Build history of the part. All positions in model axes, mm. Round coordinates to 2 decimals unless told otherwise and drop trailing zeros. Loops run counter-clockwise (first coordinate to the right, second up) from the corner with the lowest first, then second, coordinate; pieces in that order, holes last.
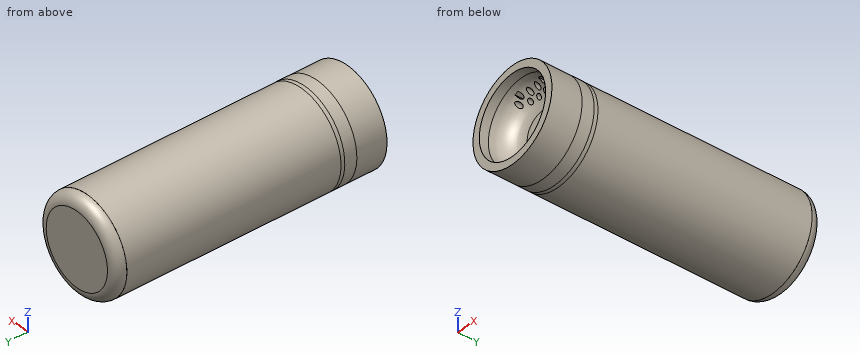
from build123d import *

# Parameters (mm, degrees)
SKETCH1_R           = 15.591175954
BOSS_EXTRUDE1_DEPTH = 71
BOSS_EXTRUDE2_START = 1.25
SKETCH2_R           = 15.591175954
SKETCH2_W           = 17.8
SKETCH2_H           = 1.65
BOSS_EXTRUDE2_DEPTH = 1.25
BOSS_EXTRUDE3_START = 4
SKETCH3_R           = 15.591175954
BOSS_EXTRUDE3_DEPTH = 4
CUT_EXTRUDE4_START  = -11.5
SKETCH16_R          = 0.75
CUT_EXTRUDE4_DEPTH  = 11.5
BOSS_EXTRUDE8_START = 10
SKETCH18_R          = 15.591175954
SKETCH18_R_2        = 13.095738675
BOSS_EXTRUDE8_DEPTH = 10
FILLET3_START       = -12.2500001
FILLET3_OUTLINE_R   = 13.095738675
FILLET3_OUTLINE_R_2 = 0.75
FILLET3_DEPTH       = 7.0000001
FILLET3_START_2     = -11
FILLET3_3_DEPTH     = 5.75
SKETCH26_R          = 15.591175954
BOSS_EXTRUDE9_DEPTH = 3.5
FILLET4_R           = 3.5


with BuildPart() as part:
    # Sketch1 → Boss-Extrude1 (new body)
    with BuildSketch(Plane(origin=(0, 0, 0), x_dir=(1, 0, 0), z_dir=(0, 1, 0))):
        with Locations(Location((0, 0, 0), (0, 0, 270))):
            Circle(SKETCH1_R)
        with BuildLine():
            Line((8.375, -6.964282891), (9.075, -6.964282891))
            Line((9.075, -6.964282891), (9.075, -8.614282891))
            Line((9.075, -8.614282891), (8.375, -8.614282891))
            Line((8.375, -8.614282891), (8.375, -9.610929808))
            ThreePointArc((8.375, -9.610929808), (0, -12.747964417), (-8.375, -9.610929808))
            Line((-8.375, -9.610929808), (-8.375, -8.614282891))
            Line((-8.375, -8.614282891), (-8.725, -8.614282891))
            Line((-8.725, -8.614282891), (-8.725, -6.964282891))
            Line((-8.725, -6.964282891), (-8.375, -6.964282891))
            Line((-8.375, -6.964282891), (-8.375, -6.204282891))
            Line((-8.375, -6.204282891), (-8.375, 9.645717109))
            ThreePointArc((-8.375, 9.645717109), (-7.386485387, 12.032202496), (-5, 13.020717109))
            Line((-5, 13.020717109), (5, 13.020717109))
            ThreePointArc((5, 13.020717109), (7.386485387, 12.032202496), (8.375, 9.645717109))
            Line((8.375, 9.645717109), (8.375, -6.204282891))
            Line((8.375, -6.204282891), (8.375, -6.964282891))
        make_face(mode=Mode.SUBTRACT)
    extrude(amount=BOSS_EXTRUDE1_DEPTH)

    # Sketch2 → Boss-Extrude2 (add)
    with BuildSketch(Plane.XZ.offset(BOSS_EXTRUDE2_START)):
        with Locations(Location((0, 0, 0), (0, 0, 270))):
            Circle(SKETCH2_R)
        with Locations((0.175, 7.789282891)):
            Rectangle(SKETCH2_W, SKETCH2_H, mode=Mode.SUBTRACT)
    extrude(amount=-BOSS_EXTRUDE2_DEPTH)

    # Sketch3 → Boss-Extrude3 (add)
    with BuildSketch(Plane.XZ.offset(1.25).offset(BOSS_EXTRUDE3_START)):
        with Locations(Location((0, 0, 0), (0, 0, 270))):
            Circle(SKETCH3_R)
    extrude(amount=-BOSS_EXTRUDE3_DEPTH)

    # Sketch16 → Cut-Extrude4 (cut)
    with BuildSketch(Plane(origin=(0, 0, 0), x_dir=(1, 0, 0), z_dir=(0, 1, 0)).offset(CUT_EXTRUDE4_START)):
        with BuildLine():
            Line((-3.75, -9.901070776), (-3, -9.901070776))
            Line((-3, -9.901070776), (-2.25, -9.901070776))
            ThreePointArc((-2.25, -9.901070776), (-3, -9.151070776), (-3.75, -9.901070776))
        make_face()
        with BuildLine():
            Line((-2.25, -9.901070776), (-3, -9.901070776))
            Line((-3, -9.901070776), (-3.75, -9.901070776))
            ThreePointArc((-3.75, -9.901070776), (-3, -10.651070776), (-2.25, -9.901070776))
        make_face()
        with BuildLine():
            ThreePointArc((6.75, -9.901070776), (6, -9.151070776), (5.25, -9.901070776))
            ThreePointArc((5.25, -9.901070776), (6, -10.651070776), (6.75, -9.901070776))
        make_face()
        with BuildLine():
            ThreePointArc((3.75, -9.901070776), (3, -9.151070776), (2.25, -9.901070776))
            Line((2.25, -9.901070776), (3, -9.901070776))
            Line((3, -9.901070776), (3.75, -9.901070776))
        make_face()
        with BuildLine():
            Line((3, -9.901070776), (2.25, -9.901070776))
            ThreePointArc((2.25, -9.901070776), (3, -10.651070776), (3.75, -9.901070776))
            Line((3.75, -9.901070776), (3, -9.901070776))
        make_face()
        with BuildLine():
            ThreePointArc((0.75, -9.901070776), (0, -9.151070776), (-0.75, -9.901070776))
            Line((-0.75, -9.901070776), (0, -9.901070776))
            Line((0, -9.901070776), (0.75, -9.901070776))
        make_face()
        with BuildLine():
            Line((0, -9.901070776), (-0.75, -9.901070776))
            ThreePointArc((-0.75, -9.901070776), (0, -10.651070776), (0.75, -9.901070776))
            Line((0.75, -9.901070776), (0, -9.901070776))
        make_face()
        with Locations(Location((-6, -9.901070776, 0), (0, 0, 270))):
            Circle(SKETCH16_R)
        with BuildLine():
            ThreePointArc((5.289192257, -11.598924176), (4.550417773, -10.824582592), (3.789595018, -11.577272013))
            ThreePointArc((3.789595018, -11.577272013), (3.846450326, -11.860961254), (4.006459728, -12.102019552))
            ThreePointArc((4.006459728, -12.102019552), (4.654628095, -11.867815051), (5.289192257, -11.598924176))
        make_face()
        with BuildLine():
            ThreePointArc((2.290136401, -11.577272013), (1.540136401, -10.827272013), (0.790136401, -11.577272013))
            Line((0.790136401, -11.577272013), (1.540136401, -11.577272013))
            Line((1.540136401, -11.577272013), (2.290136401, -11.577272013))
        make_face()
        with BuildLine():
            Line((1.540136401, -11.577272013), (0.790136401, -11.577272013))
            ThreePointArc((0.790136401, -11.577272013), (1.540136401, -12.327272013), (2.290136401, -11.577272013))
            Line((2.290136401, -11.577272013), (1.540136401, -11.577272013))
        make_face()
        with BuildLine():
            ThreePointArc((-0.707561207, -11.577133163), (-2.207561203, -11.577063737), (-0.707561219, -11.577272013))
            ThreePointArc((-0.707561219, -11.577272013), (-0.70756121, -11.577202588), (-0.707561207, -11.577133163))
        make_face()
        with BuildLine():
            ThreePointArc((-5.205190023, -11.636863564), (-4.580517042, -11.896615502), (-3.942943702, -12.122862358))
            ThreePointArc((-3.942943702, -12.122862358), (-4.188076003, -10.877359358), (-5.205190023, -11.636863564))
        make_face()
    extrude(amount=CUT_EXTRUDE4_DEPTH, mode=Mode.SUBTRACT)

    # Sketch18 → Boss-Extrude8 (add)
    with BuildSketch(Plane.XZ.offset(5.25).offset(BOSS_EXTRUDE8_START)):
        with Locations(Location((0, 0, 0), (0, 0, 270))):
            Circle(SKETCH18_R)
        with Locations(Location((0, 0, 0), (0, 0, 270))):
            Circle(SKETCH18_R_2, mode=Mode.SUBTRACT)
    extrude(amount=-BOSS_EXTRUDE8_DEPTH)

    # Fillet3: read off the stored shape, not the designer's step
    # Fillet3 outline → Fillet3 (add)
    with BuildSketch(Plane(origin=(0, 0, 0), x_dir=(1, 0, 0), z_dir=(0, 1, 0)).offset(FILLET3_START)):
        Circle(FILLET3_OUTLINE_R)
        with Locations((-6, -9.901070776)):
            Circle(FILLET3_OUTLINE_R_2, mode=Mode.SUBTRACT)
        with Locations((-1.457561207, -11.577133163)):
            Circle(FILLET3_OUTLINE_R_2, mode=Mode.SUBTRACT)
        with Locations((-3, -9.901070776)):
            Circle(FILLET3_OUTLINE_R_2, mode=Mode.SUBTRACT)
        with Locations((1.540136401, -11.577272013)):
            Circle(FILLET3_OUTLINE_R_2, mode=Mode.SUBTRACT)
        with Locations((0, -9.901070776)):
            Circle(FILLET3_OUTLINE_R_2, mode=Mode.SUBTRACT)
        with Locations((3, -9.901070776)):
            Circle(FILLET3_OUTLINE_R_2, mode=Mode.SUBTRACT)
        with Locations((6, -9.901070776)):
            Circle(FILLET3_OUTLINE_R_2, mode=Mode.SUBTRACT)
    extrude(amount=FILLET3_DEPTH)

    # Fillet3 2 outline → Fillet3 2 (revolve, cut)
    with BuildSketch(Plane.XY):
        with BuildLine():
            Line((6.095738675, -5.25), (0, -5.25))
            Line((0, -5.25), (0, -12.25))
            Line((0, -12.25), (13.095738675, -12.25))
            ThreePointArc((13.095738675, -12.25), (11.045486143, -7.300252532), (6.095738675, -5.25))
        make_face()
    revolve(axis=Axis((0, 0, 0), (0, 1, 0)), mode=Mode.SUBTRACT)

    # Fillet3 3 outline → Fillet3 3 (cut)
    with BuildSketch(Plane(origin=(0, 0, 0), x_dir=(1, 0, 0), z_dir=(0, 1, 0)).offset(FILLET3_START_2)):
        with BuildLine():
            ThreePointArc((4.006459728, -12.102019552), (4.654628094, -11.867815051), (5.289192257, -11.598924176))
            ThreePointArc((5.289192257, -11.598924176), (4.265744538, -10.876286186), (4.006459728, -12.102019552))
        make_face()
        with BuildLine():
            ThreePointArc((-5.205190023, -11.636863564), (-4.580517042, -11.896615502), (-3.942943702, -12.122862358))
            ThreePointArc((-3.942943702, -12.122862358), (-4.188076003, -10.877359358), (-5.205190023, -11.636863564))
        make_face()
    extrude(amount=FILLET3_3_DEPTH, mode=Mode.SUBTRACT)

    # Sketch26 → Boss-Extrude9 (add)
    with BuildSketch(Plane(origin=(0, 71, 0), x_dir=(1, 0, 0), z_dir=(0, 1, 0))):
        with Locations(Location((0, 0, 0), (0, 0, 90))):
            Circle(SKETCH26_R)
    extrude(amount=BOSS_EXTRUDE9_DEPTH)

    # Fillet4
    fillet4_edges = [part.edges().sort_by_distance(p)[0] for p in [
        (0, 74.5, 15.591175954),
    ]]
    fillet(fillet4_edges, radius=FILLET4_R - 0.0001)  # a hair under: the kernel refuses the full size


solid = part.part
(1) Pin check, flat tips, straight feed: P1, Ø4, axis at y = 0, z = -5, coming from the +X side; P2, Ø1.4, axis at y = -0.5, z = 7.5, coming from the -X side; P3, Ø0.5, axis at y = 24, z = 7.5, coming from the +X side. Stop position of each tip, or through.
Responses:
P1: stops at x = 15.3
P2: stops at x = -14.03
P3: stops at x = 13.8
(2) Slice it at A-A on y = 11.5. List the corners of the cut face in (x, z) (3 decimals).
Responses:
outline: circle Ø31.182 at (0, 0); hole (-8.725, 6.964) - (-8.375, 6.964) - (-8.375, -9.646) arc R3.375 ccw to (-5, -13.021) - (5, -13.021) arc R3.375 ccw to (8.375, -9.646) - (8.375, 6.964) - (9.075, 6.964) - (9.075, 8.614) - (8.375, 8.614) - (8.375, 9.611) arc R12.748 ccw to (-8.375, 9.611) - (-8.375, 8.614) - (-8.725, 8.614) - close
(3) Probe line 1 (X direction, y = -1.5, z = 9.5); line 2 (Y direction, x = 4, z = -2); line 3 (Z direction, x = -2.5, y = -7.5). List the from-to ranges inside material, lowest first.
Responses:
line 1: x = -12.36 to -6.63, -5.37 to -3.63, -2.37 to -0.63, 0.63 to 2.37, 3.63 to 5.37, 6.63 to 12.36
line 2: y = -5.25 to 0, 71 to 74.5
line 3: z = -15.39 to -10.96, 10.96 to 15.39
